```python
from build123d import *

# Parameters (mm, degrees)
F1_DEPTH = 10.31875
F2_W     = 9.525
F2_H     = 69.85
F3_DEPTH = 25.4
F4_W     = 9.525
F4_H     = 69.85
F5_DEPTH = 25.4
F6_W     = 7.9375
F6_H     = 431.8
F7_DEPTH = 9.525


with BuildPart() as f1:
    # F0 (on Right) → F1 (new body, symmetric)
    with BuildSketch(Plane.YZ):
        with BuildLine():
            Line((215.9, 44.45), (-215.9, 44.45))
            Line((-215.9, 44.45), (-215.9, -44.45))
            ThreePointArc((-215.9, -44.45), (0, -24.998684), (215.9, -44.45))
            Line((215.9, -44.45), (215.9, 44.45))
        make_face()
    extrude(amount=F1_DEPTH, both=True)

    # F2 (on face) → F3 (join)
    with BuildSketch(Plane.XZ.offset(215.9)):
        Rectangle(F2_W, F2_H)
    extrude(amount=F3_DEPTH)

    # F4 (on face) → F5 (join)
    with BuildSketch(Plane(origin=(0, 215.9, 0), x_dir=(-1, 0, 0), z_dir=(0, 1, 0))):
        Rectangle(F4_W, F4_H)
    extrude(amount=F5_DEPTH)

    # F6 (on face) → F7 (cut)
    with BuildSketch(Plane.XY.offset(44.45)):
        Rectangle(F6_W, F6_H)
    extrude(amount=-F7_DEPTH, mode=Mode.SUBTRACT)


solid = f1.part
```
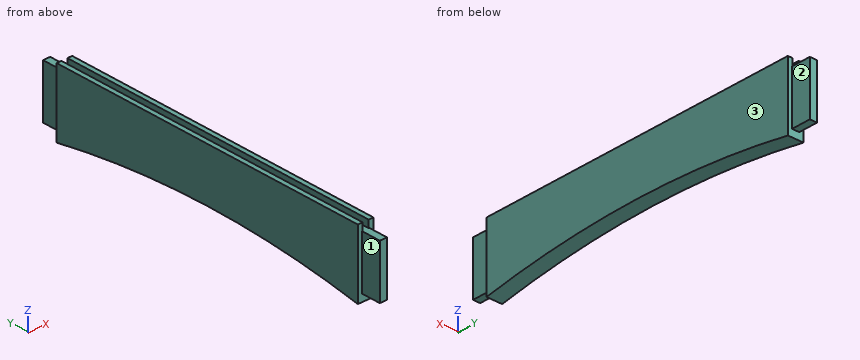
Could you check a few things on this model? Use its own coordinates, in mm. Face numbers are marked on the shaded views. A direction names the side the tool comes from. Round coordinates to 2 decimals unless told otherwise and drop trailing zeros. Loops run counter-clockwise (first coordinate to the right, second up) from the corner with the lowest first, then second, coordinate; pieces in that order, holes last. Notation, with made-up numbers: M 13,51 L 56,51 A30 cw 56,85 Z; hole C 14,0 d6. An arc over 180 degrees is marked long. Put each result on its own line as item: value.
Q1. Imagine slicing it at A-A (x = 0.5). Write out the boundary of the cut face in (y, z) (3 decimals).
Check result:
outline: M -241.3,-34.925 L -215.9,-34.925 L -215.9,-44.45 A1207.917 cw 215.9,-44.45 L 215.9,-34.925 L 241.3,-34.925 L 241.3,34.925 L -241.3,34.925 Z
Q2. Imagine slicing it at C-C (y = 0). Write out the boundary of the cut face in (x, z) (3 decimals), then the cut area to 3 significant figures.
Check result:
outline: M -10.319,-24.999 L 10.319,-24.999 L 10.319,44.45 L 3.969,44.45 L 3.969,34.925 L -3.969,34.925 L -3.969,44.45 L -10.319,44.45 Z
area: 1,360 mm2
Q3. For pin 1 (12 mm diameter, centred on x = -8, y = -161, fed in from -Z); pin 2 (5 mm diameter, centred on x = 3.5, z = 35.5, fed in from -Y); pin 3 (2 mm diameter, centred on x = 4.5, y = -192.5, fed in from -Z); pin 4 (5 mm diameter, centred on x = -1.5, y = 229, fed in from -Z) (3 decimals), each with a flat end and sliding along its axis, tell me the tip position at first contact or that it passes through.
Check result:
pin 1: z = -36.6
pin 2: y = -241.3
pin 3: z = -40.6
pin 4: z = -34.925
Q4. On a 3-axis mill with a long thin cutter (end or side, diameter ignored), from which of +Z, -Z, +X, -X, +Y, -Y can I reach the whole of each face in a straight line? I mean the marked faces 1, 2 and 3. Say none if no direction works.
Check result:
face 1: +Z, -Z, -X, -Y
face 2: +Z, -Z, +X, +Y
face 3: +Z, -Z, +X, +Y, -Y
Q5. Imagine slicing it at B-B (z = 18). Write out the boundary of the cut face in (x, y), then the cut area to 3 significant figures.
Check result:
outline: M -10.32,-215.9 L -4.76,-215.9 L -4.76,-241.3 L 4.76,-241.3 L 4.76,-215.9 L 10.32,-215.9 L 10.32,215.9 L 4.76,215.9 L 4.76,241.3 L -4.76,241.3 L -4.76,215.9 L -10.32,215.9 Z
area: 9,400 mm2
Q6. I need wall thicknesses on probe 1 along X at (y, z) = (-57.5, 39); probe 2 along Y at (x, z) = (5.75, 39.5); probe 3 along Z at (x, y) = (4, -130). Which ranges of each line are inside material? Lowest first, please.
Check result:
probe 1: -10.32 to -3.97, 3.97 to 10.32
probe 2: -215.9 to 215.9
probe 3: -32.01 to 44.45
